from build123d import *

# Parameters (mm, degrees)
F0_W      = 400
F0_H      = 400
F1_DEPTH  = 400
F2_T      = -12
F4_W      = 376
F4_H      = 11.2500011921
F5_DEPTH  = 383
F6_W      = 376
F6_H      = 176.7499988079
F7_DEPTH  = 439
F8_T      = -2.5
F9_R      = 16.4515915788
F10_DEPTH = 25


# Not quite as in the source:
# - a shell that OpenCascade refuses in one call is made with other operations: the cavity is built on its own and cut out


with BuildPart() as f1:
    # F0 (on Top) → F1 (new body)
    with BuildSketch(Plane.XY):
        with Locations((-4.0007606149, 88.9041203893)):
            Rectangle(F0_W, F0_H)
    extrude(amount=F1_DEPTH)

    # F2
    f2_openings = [f1.faces().sort_by_distance(p)[0] for p in [
        (-4.000761, -111.09588, 200),
    ]]
    offset(amount=F2_T, openings=f2_openings)

    # F4 (on face) → F5 (join)
    with BuildSketch(Plane.XZ.offset(-276.9041203893)):
        with Locations((-4.0007606149, 194.374999404)):
            Rectangle(F4_W, F4_H)
    extrude(amount=F5_DEPTH)

    # F6 (on face) → F7 (join)
    with BuildSketch(Plane.XZ.offset(-276.9041203893)):
        with Locations((-4.0007606149, 100.374999404)):
            Rectangle(F6_W, F6_H)
    extrude(amount=F7_DEPTH)

    # F8: a shell. OpenCascade refuses it in one call, so the cavity is built on its own and cut out:
    # the body offset inwards by the wall thickness, plus a prism from it out through each open face.
    f8_core = offset(f1.part, amount=F8_T, kind=Kind.INTERSECTION, mode=Mode.PRIVATE)
    f8_exits = [f8_core.faces().sort_by_distance(p)[0] for p in [
        (-4.000761, -131.534658, 186.249999),
    ]]
    add(f8_core, mode=Mode.SUBTRACT)
    extrude(f8_exits, amount=-F8_T, mode=Mode.SUBTRACT)

    # F9 (on face) → F10 (join)
    with BuildSketch(Plane.XZ.offset(162.0958796107)):
        with Locations((-22.2093164921, 107.9253256321)):
            Circle(F9_R)
    extrude(amount=F10_DEPTH)


solid = f1.part
Design review of the part built by this model. Coordinates are the model's own, in mm. A direction names the side the tool comes from. Coordinates: 2 decimals unless noted, no trailing zeros. Order: outer loops, then holes, each group sorted by start corner. A loop starts at its lowest first (then second) coordinate and runs counter-clockwise, first axis right, second up.
Item 1: For faces 5 (the flat face through (-192.001, -136, 99)), 6 (the flat face through (-7, -136, 12)), 7 (the flat face through (-7, 86, 388)), 8 (the flat face through (-7, -159.596, 100)), 9 (the flat face through (193.499, 86, 197)), list the 3-axis set-ups (+Z, -Z, +X, -X, +Y, -Y) from which the entire face can be reached by the end or side of a thin tool; tool diameter is ignored.
Item 2: For pin 1 Ø1.5 at (x, z) = (6.5, 172) entering from -Y; pin 2 Ø5 at (x, z) = (-39.5, 257.5) entering from -Y, all flat-tipped, find the tip position at first contact; note any pin that passes through.
Item 3: For line 1 (Z direction, x = 43.5, y = -86); line 2 (X direction, y = -15.5, z = 201); line 3 (X direction, y = -50, z = 17), list the stretches that pass through material, from the lowest coordinate up.
Item 4: Take a section at A-A, the plane y = 246. Write out the cut boundary in (x, z), then the cut area to 3 significant figures.
Item 5: Take a section at C-C, the plane x = 1.5. Write out the cut boundary in (y, z), then the cut area to 3 significant figures.
Item 6: Take a section at B-B, the plane z = 131.5. Write out the cut boundary in (x, y), then the cut area to 3 significant figures.
Item 7: The part is to be moulded in two halves that separate along Y. For faces 1 (the flat face through (-7, 92, 2.5)), 2 (the flat face through (-7, 276.904, 293)), 3 (the flat face through (183.999, -136, 99)), 4 (the flat face through (-7, 91, 197.5)), say which applies: pulls with the +Y half, pulls with the -Y half, needs draft (parallel to the pull), parting line crosses it, or undercut.
Item 8: Take a section at D-D, the plane y = -129. Write out the cut boundary in (x, z).
The answers:
1. face 5: +Z, -Z, -X, -Y
1. face 6: -Z, +X, -X, -Y
1. face 7: -Y
1. face 8: +Z
1. face 9: none
2. pin 1: stops at y = -162.1
2. pin 2: stops at y = 276.9
3. line 1: z = 0 to 2.5, 197.5 to 200, 388 to 390.5, 397.5 to 400
3. line 2: x = -204 to -201.5, -194.5 to -192, 184 to 186.5, 193.5 to 196
3. line 3: x = -204 to -201.5, 193.5 to 196
4. outline: (-204, 0) - (196, 0) - (196, 400) - (-204, 400) - close; (-194.5, 197.5) - (186.5, 197.5) - (186.5, 390.5) - (-194.5, 390.5) - close; hole (-201.5, 2.5) - (193.5, 2.5) - (193.5, 397.5) - (-201.5, 397.5) - close; hole (-192, 200) - (184, 200) - (184, 388) - (-192, 388) - close
4. area: 6,820 mm2
5. outline: (-162.1, 12) - (-111.1, 12) - (-111.1, 0) - (288.9, 0) - (288.9, 400) - (-111.1, 400) - (-111.1, 388) - (276.9, 388) - (276.9, 200) - (-106.1, 200) - (-106.1, 188.75) - (-103.6, 188.75) - (-103.6, 197.5) - (279.4, 197.5) - (279.4, 390.5) - (-108.6, 390.5) - (-108.6, 397.5) - (286.4, 397.5) - (286.4, 2.5) - (-108.6, 2.5) - (-108.6, 14.5) - (-159.6, 14.5) - (-159.6, 188.75) - (-162.1, 188.75) - close
5. area: 6,030 mm2
6. outline: (-204, -111.1) - (-192, -111.1) - (-192, -162.1) - (184, -162.1) - (184, -111.1) - (196, -111.1) - (196, 288.9) - (-204, 288.9) - close; hole (-201.5, -108.6) - (-189.5, -108.6) - (-189.5, -159.6) - (181.5, -159.6) - (181.5, -108.6) - (193.5, -108.6) - (193.5, 286.4) - (-201.5, 286.4) - close
6. area: 4,230 mm2
7. face 1: undercut
7. face 2: pulls with the -Y half
7. face 3: needs draft
7. face 4: undercut
8. outline: (-192, 12) - (184, 12) - (184, 188.75) - (181.5, 188.75) - (181.5, 14.5) - (-189.5, 14.5) - (-189.5, 188.75) - (-192, 188.75) - close
